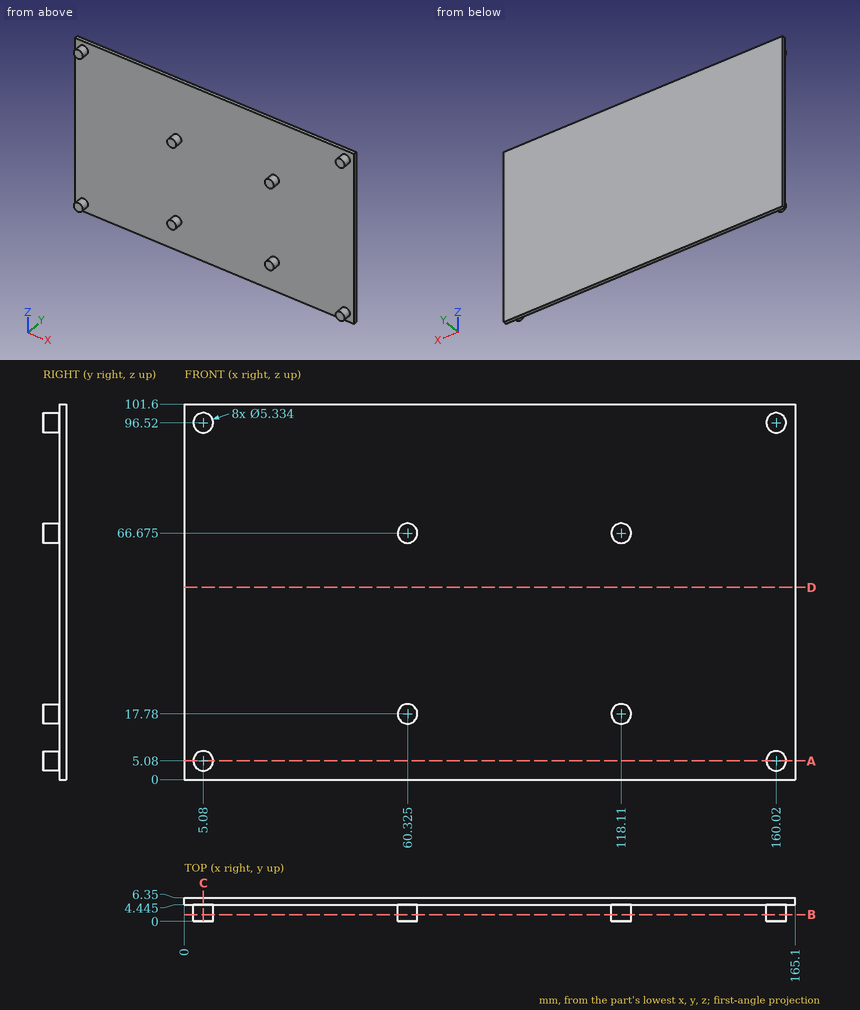
Verification items for this drawing (mm, ordinates from the low corner). Coordinates: 2 decimals unless noted, no trailing zeros. Loops run counter-clockwise (first coordinate to the right, second up) from the corner with the lowest first, then second, coordinate; pieces in that order, holes last. Notation, with made-up numbers: (-16, 26) - (19, 26) arc R18 cw to (19, 39) - close; hole circle Ø11 at (69.25, 72.5). An arc over 180 degrees is marked (long way). Answer as a JSON object with one key per item and string values.
(1) Cross-section at D-D, the plane z = 52. Record the boundary of the cut face in (x, y) (3 decimals).
Response:
{"outline": "(0, 4.445) - (165.1, 4.445) - (165.1, 6.35) - (0, 6.35) - close"}
(2) Cross-section at A-A, the plane z = 5.08. Record the boundary of the cut face in (x, y) (3 decimals), then the cut area to 3 significant figures.
Response:
{"outline": "(0, 4.445) - (2.413, 4.445) - (2.413, 0) - (7.747, 0) - (7.747, 4.445) - (157.353, 4.445) - (157.353, 0) - (162.687, 0) - (162.687, 4.445) - (165.1, 4.445) - (165.1, 6.35) - (0, 6.35) - close", "area": "362 mm²"}
(3) Scan line: line 1 along Y through (x, z) = (112, 7) (3 decimals). Record every from-to range of solid material in increasing order.
Response:
{"line 1": "y = 4.445 to 6.35"}
(4) Cross-section at B-B, the plane y = 1.75. Record the boundary of the cut face in (x, z) (3 decimals).
Response:
{"outline": "circle Ø5.334 at (5.08, 5.08); circle Ø5.334 at (5.08, 96.52); circle Ø5.334 at (60.325, 17.78); circle Ø5.334 at (60.325, 66.675); circle Ø5.334 at (118.11, 17.78); circle Ø5.334 at (118.11, 66.675); circle Ø5.334 at (160.02, 5.08); circle Ø5.334 at (160.02, 96.52)"}
(5) Cross-section at C-C, the plane x = 5.08. Record the boundary of the cut face in (y, z) (3 decimals).
Response:
{"outline": "(0, 2.413) - (4.445, 2.413) - (4.445, 0) - (6.35, 0) - (6.35, 101.6) - (4.445, 101.6) - (4.445, 99.187) - (0, 99.187) - (0, 93.853) - (4.445, 93.853) - (4.445, 7.747) - (0, 7.747) - close"}
(6) Go/stop test with flat-tipped pins: pin 1 Ø1 at (x, z) = (63, 54.5) entering from -Y (3 decimals); pin 2 Ø1 at (x, y) = (66, 3.5) entering from +Z; pin 3 Ø3 at (y, z) = (5.5, 79.5) entering from -X. Record where each tip stops, or that it passes through.
Response:
{"pin 1": "stops at y = 4.445", "pin 2": "passes through", "pin 3": "stops at x = 0"}
